from build123d import *

# Parameters (mm, degrees)
SKETCH2_R           = 25
SKETCH2_R_2         = 23
BOSS_EXTRUDE1_DEPTH = 320
BOSS_EXTRUDE2_START = 54
SKETCH2_3_R         = 26
SKETCH2_3_R_2       = 25
BOSS_EXTRUDE2_DEPTH = 4
SKETCH2_4_R         = 26
SKETCH2_4_R_2       = 25
BOSS_EXTRUDE3_DEPTH = 4


with BuildPart() as part:
    # Sketch2 → Boss-Extrude1 (new body)
    with BuildSketch(Plane.XY):
        Circle(SKETCH2_R)
        Circle(SKETCH2_R_2, mode=Mode.SUBTRACT)
    extrude(amount=BOSS_EXTRUDE1_DEPTH)

    # Sketch2<3> → Boss-Extrude2 (add)
    with BuildSketch(Plane.XY.offset(BOSS_EXTRUDE2_START)):
        Circle(SKETCH2_3_R)
        Circle(SKETCH2_3_R_2, mode=Mode.SUBTRACT)
    extrude(amount=BOSS_EXTRUDE2_DEPTH)

    # Sketch2<4> → Boss-Extrude3 (add)
    with BuildSketch(Plane.XY):
        Circle(SKETCH2_4_R)
        Circle(SKETCH2_4_R_2, mode=Mode.SUBTRACT)
    extrude(amount=BOSS_EXTRUDE3_DEPTH)


solid = part.part
Could you check a few things on this model? Use its own coordinates, in mm. A direction names the side the tool comes from. Give positions to 0.01 mm unless a question says otherwise; leave off trailing zeros. Order: outer loops, then holes, each group sorted by start corner. A loop starts at its lowest first (then second) coordinate and runs counter-clockwise, first axis right, second up. Notation, with made-up numbers: (56, 36.25) - (105, 36.25) arc R27 ccw to (105, 52.25) - close; hole circle Ø1 at (-27, -15). An arc over 180 degrees is marked (long way). One line per question, with ' | ' between items. Start each with the question number.
Item 1: I need wall thicknesses on probe 1 along Y at (x, z) = (0, 91); probe 2 along X at (y, z) = (-0.5, 88.5) (3 decimals); probe 3 along Y at (x, z) = (-17.5, 305.5). Which ranges of each line are inside material? Lowest first, please. Write a range as [from, to].
Item 2: I want a section at C-C on z = 112.5. Write out the boundary of the cut face in (x, y), then the cut area to 3 significant figures.
Item 3: I want a section at A-A on y = 0. Write out the boundary of the cut face in (x, z), then the cut area to 3 significant figures.
Item 4: I'm going to push flat-ended pins straight in: pin 1 Ø12 at (x, z) = (3, 140.5) entering from -Y; pin 2 Ø5 at (x, z) = (-7.5, 237) entering from -Y; pin 3 Ø5 at (x, z) = (-8, 117) entering from +Y. Where does each tip first touch, or does it pass through?
Item 5: For faces 5 (the flat face through (22.1, -7.3, 320)), 6 (the flat face through (-14, 21, 58)), 7 (the flat face through (-14, 21, 4)), which set-ups out of +Z, -Z, +X, -X, +Y, -Y let a thin tool reach every point of the face, with its end or its side?
Item 6: Thinking about a two-plate mould opening in Z: for faces 1 (the cylindrical face through (23.846, 7.509, 187.166)), 2 (the flat face through (10, -21, 0)), 3 (the flat face through (-14, 21, 54)), 4 (the cylindrical face through (23.846, 7.509, 28.65)), which applies, pulls with the +Z half, pulls with the -Z half, needs draft (parallel to the pull), parting line crosses it, or undercut?
Verdict:
1) probe 1: [-25, -23], [23, 25] | probe 2: [-24.995, -22.995], [22.995, 24.995] | probe 3: [-17.85, -14.92], [14.92, 17.85]
2) outline: circle Ø50 at (0, 0); hole circle Ø46 at (0, 0) | area: 302 mm^2
3) outline: (-26, 0) - (-23, 0) - (-23, 320) - (-25, 320) - (-25, 58) - (-26, 58) - (-26, 54) - (-25, 54) - (-25, 4) - (-26, 4) - close; (23, 0) - (26, 0) - (26, 4) - (25, 4) - (25, 54) - (26, 54) - (26, 58) - (25, 58) - (25, 320) - (23, 320) - close | area: 1,300 mm^2
4) pin 1: y = -25 | pin 2: y = -24.49 | pin 3: y = 24.39
5) face 5: +Z, +X, -X, +Y, -Y | face 6: +Z | face 7: none
6) face 1: needs draft | face 2: pulls with the -Z half | face 3: undercut | face 4: undercut
